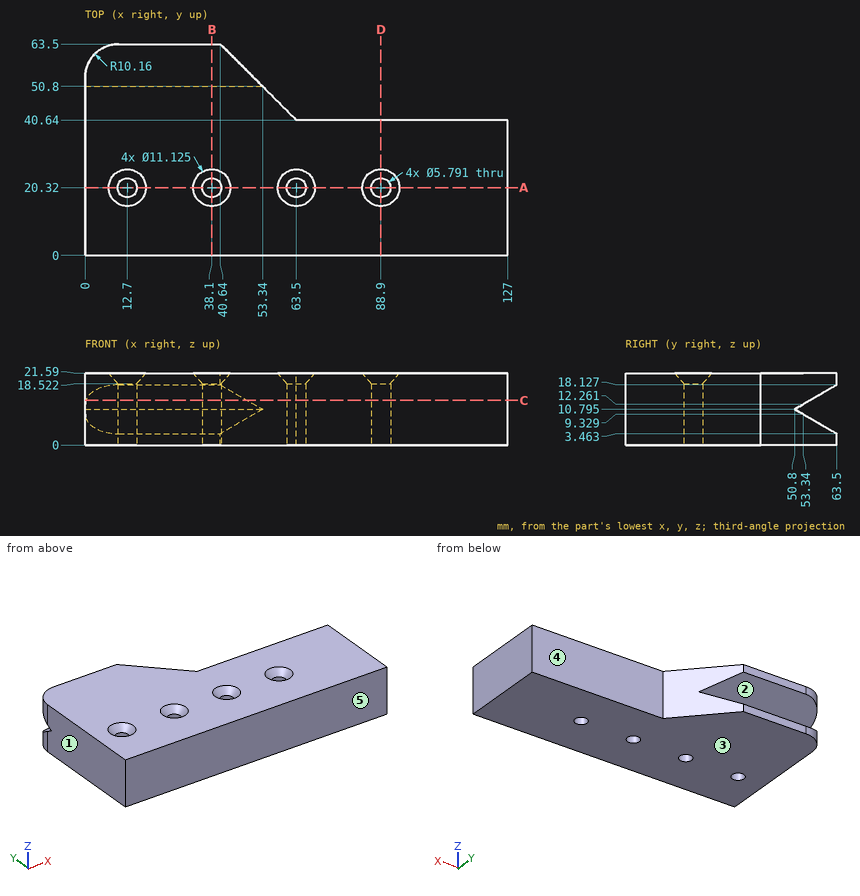
Input: dimensioned drawing with shaded views. Units: mm. Origin: part minimum x, y, z. A direction names the side the tool comes from. Give positions to 0.01 mm unless a question says otherwise; leave off trailing zeros. Order: outer loops, then holes, each group sorted by start corner. A loop starts at its lowest first (then second) coordinate and runs counter-clockwise, first axis right, second up. Notation, with made-up numbers: (31, 21.25) -> (72, 21.25) arc R20 cw to (72, 55.25) -> close; hole circle Ø5 at (46, 72.5). An arc over 180 degrees is marked (long way). Use one line per item in the form item = value.
1) First-contact query: pin 1 Ø3.5 at (x, y) = (38.1, 20.32) entering from +Z; pin 2 Ø11 at (x, z) = (87.5, 15.5) entering from +Y; pin 3 Ø4 at (y, z) = (52, 13.5) entering from +X; pin 4 Ø9.5 at (x, y) = (88.9, 20.32) entering from +Z (1 decimal). Flat tips, straight axial feed; report the tip coordinate or a pass-through.
Response values:
pin_1 = through
pin_2 = 40.64
pin_3 = 54.14
pin_4 = 20.7
2) Mould query, pull axis Z, two halves, no side actions, for the marked faces 1, 2 and 3. Classes: pulls with the +Z half, pulls with the -Z half, needs draft (parallel to the pull), parting line crosses it, or undercut.
Response values:
face_1 = needs draft
face_2 = undercut
face_3 = pulls with the -Z half
3) Reachability of the marked faces 4 and 5 from +Z, -Z, +X, -X, +Y, -Y: full face, straight path, thin tool, end or side. Return the list, or none.
Response values:
face_4 = +Z, -Z, +X, +Y
face_5 = +Z, -Z, +X, -X, -Y
4) Section C-C, the plane z = 13.5. Return loops of the section in (x, y) (1 decimal), and give its area (3 significant figures).
Response values:
outline = (0, 0) -> (127, 0) -> (127, 40.6) -> (63.5, 40.6) -> (48.7, 55.5) -> (0.2, 55.5) arc R10.2 ccw to (0, 53.3) -> close; hole circle Ø5.8 at (12.7, 20.3); hole circle Ø5.8 at (38.1, 20.3); hole circle Ø5.8 at (63.5, 20.3); hole circle Ø5.8 at (88.9, 20.3)
area = 5,890 mm^2
5) Section A-A, the plane y = 20.32. Return loops of the section in (x, z) (1 decimal), and give its area (3 significant figures).
Response values:
outline = (0, 0) -> (9.8, 0) -> (9.8, 18.5) -> (7.1, 21.6) -> (0, 21.6) -> close; (15.6, 0) -> (35.2, 0) -> (35.2, 18.5) -> (32.5, 21.6) -> (18.3, 21.6) -> (15.6, 18.5) -> close; (41, 0) -> (60.6, 0) -> (60.6, 18.5) -> (57.9, 21.6) -> (43.7, 21.6) -> (41, 18.5) -> close; (66.4, 0) -> (86, 0) -> (86, 18.5) -> (83.3, 21.6) -> (69.1, 21.6) -> (66.4, 18.5) -> close; (91.8, 0) -> (127, 0) -> (127, 21.6) -> (94.5, 21.6) -> (91.8, 18.5) -> close
area = 2,210 mm^2
6) Section D-D, the plane x = 88.9. Return loops of the section in (y, z) (1 decimal).
Response values:
outline = (0, 0) -> (17.4, 0) -> (17.4, 18.5) -> (14.8, 21.6) -> (0, 21.6) -> close; (23.2, 0) -> (40.6, 0) -> (40.6, 21.6) -> (25.9, 21.6) -> (23.2, 18.5) -> close
7) Section B-B, the plane x = 38.1. Return loops of the section in (y, z) (1 decimal), and give its area (3 significant figures).
Response values:
outline = (0, 0) -> (17.4, 0) -> (17.4, 18.5) -> (14.8, 21.6) -> (0, 21.6) -> close; (23.2, 0) -> (63.5, 0) -> (63.5, 3.5) -> (50.8, 10.8) -> (63.5, 18.1) -> (63.5, 21.6) -> (25.9, 21.6) -> (23.2, 18.5) -> close
area = 1,140 mm^2
8) Line query: probe 1 along X at (y, z) = (20.32, 4.5) (1 decimal); probe 2 along Y at (x, z) = (88.9, 13.25) (1 decimal); probe 3 along X at (y, z) = (22, 12.25). Output: solid intervals per line, ascending.
Response values:
probe_1 = 0 to 9.8, 15.6 to 35.2, 41 to 60.6, 66.4 to 86, 91.8 to 127
probe_2 = 0 to 17.4, 23.2 to 40.6
probe_3 = 0 to 10.34, 15.06 to 35.74, 40.46 to 61.14, 65.86 to 86.54, 91.26 to 127
